The model under review builds one solid part; all positions refer to its coordinate system, in mm. Round coordinates to 2 decimals unless told otherwise and drop trailing zeros. Write each loop counter-clockwise with the first axis right and the second up, starting at its lowest first coordinate (ties: lowest second). Pieces come first, ordered by that corner, then holes. Notation, with made-up numbers: (52.25, 55.25) -> (84.25, 55.25) arc R23 cw to (84.25, 78.25) -> close; hole circle Ø6 at (31.5, 51.5). An arc over 180 degrees is marked (long way). Answer as a JSON object with one key per item and string values. Group by question number.
1) We need section A-A, the plane y = 5. Write out the cut boundary in (x, z), then the cut area to 3 significant figures.
2) To check wall thickness, follow probe 1 along Y at (x, z) = (55, 1.5). State the ranges of the line that lie inside material, in increasing order. Write a range as [from, to].
3) Insertion check: pin 1 Ø6 at (x, y) = (51, 20) entering from -Z; pin 2 Ø1.9 at (x, y) = (5, 5) entering from +Z. Each pin has a flat end and moves straight along its axis. Give the tip position at first contact, or say it passes through.
4) We need section B-B, the plane x = 55. Write out the cut boundary in (y, z).
from build123d import *

# Parameters (mm, degrees)
SKETCH1_W                = 60
SKETCH1_H                = 60
BOSS_EXTRUDE1_DEPTH      = 2
M3_CLEARANCE_HOLE1_D     = 3.2
M3_CLEARANCE_HOLE1_DEPTH = 2


with BuildPart() as part:
    # Sketch1 → Boss-Extrude1 (new body)
    with BuildSketch(Plane.XY):
        with Locations((30, 30)):
            Rectangle(SKETCH1_W, SKETCH1_H)
    extrude(amount=BOSS_EXTRUDE1_DEPTH)

    # M3 Clearance Hole1
    with Locations(Plane(origin=(0, 0, 0), x_dir=(-1, 0, 0), z_dir=(0, 0, -1))):
        with Locations((-55, 5), (-5, 5)):
            Hole(M3_CLEARANCE_HOLE1_D / 2, depth=M3_CLEARANCE_HOLE1_DEPTH)


solid = part.part
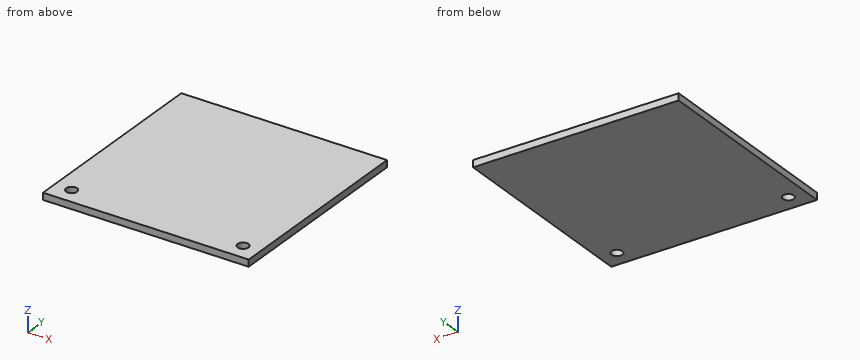
Here are the results:
{
 "1": {"outline": "(0, 0) -> (3.4, 0) -> (3.4, 2) -> (0, 2) -> close; (6.6, 0) -> (53.4, 0) -> (53.4, 2) -> (6.6, 2) -> close; (56.6, 0) -> (60, 0) -> (60, 2) -> (56.6, 2) -> close", "area": "107 mm^2"},
 "2": {"probe 1": "y = [0, 3.4], [6.6, 60]"},
 "3": {"pin 1": "stops at z = 0", "pin 2": "passes through"},
 "4": {"outline": "(0, 0) -> (3.4, 0) -> (3.4, 2) -> (0, 2) -> close; (6.6, 0) -> (60, 0) -> (60, 2) -> (6.6, 2) -> close"}
}
